from build123d import *

# Parameters (mm, degrees)
F0_W     = 288
F0_H     = 288
F0_R     = 116.5
F1_DEPTH = 288
F2_R     = 10
F4_W     = 25
F4_H     = 20
F5_DEPTH = 166.5
F7_W     = 25
F7_H     = 20
F8_DEPTH = 166.5


with BuildPart() as f1:
    # F0 (on Top) → F1 (new body)
    with BuildSketch(Plane.XY):
        Rectangle(F0_W, F0_H)
        Circle(F0_R, mode=Mode.SUBTRACT)
    extrude(amount=F1_DEPTH)

    # F2
    f2_edges = [f1.edges().sort_by_distance(p)[0] for p in [
        (144, 0, 288),
        (0, 144, 288),
        (-144, 0, 288),
        (0, -144, 288),
        (-116.5, 0, 288),
        (144, 0, 0),
        (0, 144, 0),
        (-144, 0, 0),
        (0, -144, 0),
        (-116.5, 0, 0),
        (-144, 144, 144),
        (-144, -144, 144),
        (144, -144, 144),
        (144, 144, 144),
    ]]
    fillet(f2_edges, radius=F2_R)

    # F4 (on face) → F5 (cut, symmetric)
    with BuildSketch(Plane(origin=(0, 0, 0), x_dir=(-0.7071067812, 0.7071067812, 0), z_dir=(0.7071067812, 0.7071067812, 0))):
        with Locations((0, 248)):
            Rectangle(F4_W, F4_H)
        with Locations((0, 208)):
            Rectangle(F4_W, F4_H)
    extrude(amount=F5_DEPTH, both=True, mode=Mode.SUBTRACT)

    # F7 (on face) → F8 (cut, symmetric)
    with BuildSketch(Plane(origin=(0, 0, 0), x_dir=(0.7071067812, 0.7071067812, 0), z_dir=(0.7071067812, -0.7071067812, 0))):
        with Locations((0, 248)):
            Rectangle(F7_W, F7_H)
        with Locations((0, 208)):
            Rectangle(F7_W, F7_H)
    extrude(amount=F8_DEPTH, both=True, mode=Mode.SUBTRACT)


solid = f1.part
Geometry check sheet. Reference: the model listing, model coordinates, mm. A direction names the side the tool comes from. Round coordinates to 2 decimals unless told otherwise and drop trailing zeros. Order: outer loops, then holes, each group sorted by start corner. A loop starts at its lowest first (then second) coordinate and runs counter-clockwise, first axis right, second up. Notation, with made-up numbers: M -2.75,-3 L 51.25,-3 A25 cw 51.25,35 Z; hole C 11,71.25 d3. An arc over 180 degrees is marked long. Answer in a Markdown table with one row per item.
(1) Draft check along Z on faces 1 (the face through (100, -100, 198)), 2 (the face through (1.88, 141.15, 3.01)), 3 (the face through (1.88, -141.15, 284.99)). Enter one of: released by +Z, released by -Z, zero draft, split by the parting line, or undercut.
Responses:
| item | result |
|---|---|
| face 1 | undercut |
| face 2 | released by -Z |
| face 3 | released by +Z |
(2) Sectioned sample at C-C, the plane z = 174. Record the cut outline in (x, y), and give its area (3 significant figures).
Responses:
| item | result |
|---|---|
| outline | M -144,-134 A10 ccw -134,-144 L 134,-144 A10 ccw 144,-134 L 144,134 A10 ccw 134,144 L -134,144 A10 ccw -144,134 Z; hole C 0,0 d233 |
| area | 40,200 mm² |
(3) Sectioned sample at A-A, the plane x = 0. Record the cut outline in (y, z).
Responses:
| item | result |
|---|---|
| outline | M -144,10 A10 ccw -134,0 L -126.5,0 A10 ccw -116.5,10 L -116.5,278 A10 ccw -126.5,288 L -134,288 A10 ccw -144,278 Z; M 116.5,10 A10 ccw 126.5,0 L 134,0 A10 ccw 144,10 L 144,278 A10 ccw 134,288 L 126.5,288 A10 ccw 116.5,278 Z |
(4) Tool access check on faces 4 (the face through (-117.857, 117.61, 248.14)), 5 (the face through (107.616, -44.62, 142.124)). Record the directions out of +Z, -Z, +X, -X, +Y, -Y that give a thin tool (end or side, any length) a straight path to the whole face; none if there is none.
Responses:
| item | result |
|---|---|
| face 4 | none |
| face 5 | +Z, -Z |
(5) Scan lines: probe 1 along Z at (x, y) = (-107.5, -96.5); probe 2 along Y at (x, z) = (0, 107); probe 3 along Z at (x, y) = (-84.5, 87). Record each from-to range of solid material in increasing order. Write a range as from..to.
Responses:
| item | result |
|---|---|
| probe 1 | z = 0..198, 218..238, 258..288 |
| probe 2 | y = -144..-116.5, 116.5..144 |
| probe 3 | z = 1.47..198, 218..238, 258..286.53 |
